```python
from build123d import *

# Parameters (mm, degrees)
SKETCH2_W               = 177.8
SKETCH2_H               = 101.6
SKETCH2_W_2             = 162.8
SKETCH2_H_2             = 86.6
BOSS_EXTRUDE2_DEPTH     = 2600
SKETCH1_R               = 38.1
BOSS_EXTRUDE3_DEPTH     = 44.45
BOSS_EXTRUDE5_START     = -44.45
SKETCH3_R               = 38.1
BOSS_EXTRUDE5_DEPTH     = 44.45
FILLET1_R               = 12.7
FILLET2_R               = 12.7
SKETCH5_R               = 12.7
BOSS_EXTRUDE7_DEPTH     = 19.05
CUT_EXTRUDE1_DEPTH      = 34.45
CUT_EXTRUDE2_DEPTH      = 2620.044665999
CUT_EXTRUDE2_DEPTH_BACK = 2620.044665999
SKETCH9_W               = 88.9
SKETCH9_H               = 2600


with BuildPart() as part:
    # Sketch2 → Boss-Extrude2 (new body)
    with BuildSketch(Plane.XY):
        with Locations((-88.9, 50.8)):
            Rectangle(SKETCH2_W, SKETCH2_H)
        with Locations((-88.9, 50.8)):
            Rectangle(SKETCH2_W_2, SKETCH2_H_2, mode=Mode.SUBTRACT)
    extrude(amount=BOSS_EXTRUDE2_DEPTH)

    # Sketch1 → Boss-Extrude3 (add)
    with BuildSketch(Plane(origin=(0, 0, 0), x_dir=(0, 0, -1), z_dir=(1, 0, 0))):
        with BuildLine():
            Line((-127, 101.6), (0, 101.6))
            Line((0, 101.6), (0, 304.8))
            ThreePointArc((0, 304.8), (-55.382017361, 361.922646449), (-114.190611982, 308.334272869))
            Line((-114.190611982, 308.334272869), (-127, 101.6))
        make_face()
        with Locations((-57.15, 304.8)):
            Circle(SKETCH1_R, mode=Mode.SUBTRACT)
    extrude(amount=-BOSS_EXTRUDE3_DEPTH)

    # Sketch3 → Boss-Extrude5 (add)
    with BuildSketch(Plane.ZY.offset(177.8).offset(BOSS_EXTRUDE5_START)):
        with BuildLine():
            Line((0, 304.8), (0, 101.6))
            Line((0, 101.6), (127, 101.6))
            Line((127, 101.6), (114.190611982, 308.334272869))
            ThreePointArc((114.190611982, 308.334272869), (55.382017361, 361.922646449), (0, 304.8))
        make_face()
        with Locations(Location((57.15, 304.8, 0), (0, 0, 180))):
            Circle(SKETCH3_R, mode=Mode.SUBTRACT)
    extrude(amount=BOSS_EXTRUDE5_DEPTH)

    # Fillet1
    fillet1_edges = [part.edges().sort_by_distance(p)[0] for p in [
        (-7.5, 94.1, 1300),
        (-170.3, 94.1, 1300),
        (-170.3, 7.5, 1300),
        (-7.5, 7.5, 1300),
    ]]
    fillet(fillet1_edges, radius=FILLET1_R)

    # Fillet2
    fillet2_edges = [part.edges().sort_by_distance(p)[0] for p in [
        (-44.45, 101.6, 63.5),
        (-22.225, 101.6, 127),
        (-133.35, 101.6, 63.5),
        (-155.575, 101.6, 127),
    ]]
    fillet(fillet2_edges, radius=FILLET2_R)

    # Sketch5 → Boss-Extrude7 (add)
    with BuildSketch(Plane(origin=(0, 0, 0), x_dir=(0, 0, -1), z_dir=(1, 0, 0))):
        with BuildLine():
            Line((-2600, 101.6), (-2600, 180.34))
            ThreePointArc((-2600, 180.34), (-2583.812295525, 199.173740052), (-2562.760129729, 185.999604185))
            Line((-2562.760129729, 185.999604185), (-2536.5, 101.6))
            Line((-2536.5, 101.6), (-2600, 101.6))
        make_face()
        with Locations((-2580.95, 180.34)):
            Circle(SKETCH5_R, mode=Mode.SUBTRACT)
    boss_extrude7 = extrude(amount=-BOSS_EXTRUDE7_DEPTH)

    # Mirror1: Boss-Extrude7 across plane
    add(boss_extrude7.mirror(Plane.ZY.offset(88.9)))

    # Sketch8 → Cut-Extrude1 (cut)
    with BuildSketch(Plane(origin=(-133.35, 0, 0), x_dir=(0, 0, -1), z_dir=(1, 0, 0))):
        with BuildLine():
            ThreePointArc((-10, 255.662565187), (-59.256729969, 236.73259452), (-107.248511945, 258.672469165))
            Line((-107.248511945, 258.672469165), (-115.574316238, 124.3))
            Line((-115.574316238, 124.3), (-10, 124.3))
            Line((-10, 124.3), (-10, 255.662565187))
        make_face()
    extrude(amount=-CUT_EXTRUDE1_DEPTH, mode=Mode.SUBTRACT)

    # Sketch9 → Cut-Extrude2 (cut, two sides: drawn at the far end of the back side and taken through both)
    with BuildSketch(Plane(origin=(0, 101.6, 0), x_dir=(1, 0, 0), z_dir=(0, 1, 0)).offset(-CUT_EXTRUDE2_DEPTH_BACK)):
        with Locations((-44.45, -1300)):
            Rectangle(SKETCH9_W, SKETCH9_H)
    extrude(amount=CUT_EXTRUDE2_DEPTH + CUT_EXTRUDE2_DEPTH_BACK, mode=Mode.SUBTRACT)

    # Mirror2: part across plane


with BuildPart() as part_1:
    add(part.part)
    add(part.part.mirror(Plane.ZY.offset(88.9)))


solid = part_1.part
```
Input: part model. Units: mm. Frame: model coordinates. A direction names the side the tool comes from. Round coordinates to 2 decimals unless told otherwise and drop trailing zeros. Write each loop counter-clockwise with the first axis right and the second up, starting at its lowest first coordinate (ties: lowest second). Pieces come first, ordered by that corner, then holes. Notation, with made-up numbers: (-10.75, 51.5) -> (20.25, 51.5) arc R12 ccw to (20.25, 73.5) -> close; hole circle Ø8 at (39, -17.75). An arc over 180 degrees is marked (long way). Answer as CSV lines item,"result".
1. Reachability of faces 1 (the flat face through (-155.25, 209.56, 120.31)), 2 (the flat face through (-158.75, 140, 2575)), 3 (the flat face through (-167.8, 177, 64)) from +Z, -Z, +X, -X, +Y, -Y: full face, straight path, thin tool, end or side. Return the list, or none.
Geometry says:
face 1,"+X, -X, +Y"
face 2,"+Z, +Y"
face 3,"none"
2. Section B-B (x = -89.5). Return the cut outline in (y, z).
Geometry says:
outline,"(0, 0) -> (7.5, 0) -> (7.5, 2600) -> (0, 2600) -> close; (94.1, 0) -> (101.6, 0) -> (101.6, 2600) -> (94.1, 2600) -> close"
3. Ray query, L1, parallel to X at y = 49, z = 1189; L2, parallel to Y at x = -29, z = 57.15; L3, parallel to Y at x = -91.5, z = 2159. Return the intervals inside material, ascending. Write a range as [from, to].
Geometry says:
L1,"x = [-177.8, -170.3], [-7.5, 0]"
L2,"y = [0, 7.5], [94.1, 124.3], [236.7, 266.7], [342.9, 361.95]"
L3,"y = [0, 7.5], [94.1, 101.6]"
4. Section C-C (z = 1681). Return the cut outline in (x, y), plus the area to 3 significant figures.
Geometry says:
outline,"(-177.8, 0) -> (0, 0) -> (0, 101.6) -> (-177.8, 101.6) -> close; hole (-170.3, 20.2) arc R12.7 ccw to (-157.6, 7.5) -> (-20.2, 7.5) arc R12.7 ccw to (-7.5, 20.2) -> (-7.5, 81.4) arc R12.7 ccw to (-20.2, 94.1) -> (-157.6, 94.1) arc R12.7 ccw to (-170.3, 81.4) -> close"
area,"4,100 mm^2"
5. Contact query for flat-ended pins moving along their axis: P1, Ø17, axis at x = -22.5, y = 196, coming from the +Z side; P2, Ø1.5, axis at x = -137, z = 1050.5, coming from the +Y side; P3, Ø17, axis at x = -149.5, y = 170.5, coming from the +Z side; P4, Ø4, axis at x = -99, z = 1779, coming from the -Y side. Output: stop coordinate, or through.
Geometry says:
P1,"stops at z = 2598.29"
P2,"stops at y = 101.6"
P3,"stops at z = 123.26"
P4,"stops at y = 0"
6. Mould query, pull axis X, two halves, no side actions, for faces 4 (the cylindrical face through (-22.536, 361.947, 56.614)), 5 (the flat face through (0, 61, 1198)), 6 (the flat face through (-88, 94.1, 1282)). Classes: +X half, -X half, draft (parallel to the pull), parting line (faces both ways), or undercut.
Geometry says:
face 4,"draft"
face 5,"+X half"
face 6,"undercut"
7. Section A-A (z = 57.15). Give the number of separate pieces and of enclosed holes in the cut face, plus the area to 3 significant figures.
Geometry says:
separate pieces,"3"
enclosed holes,"1"
area,"12,800 mm^2"
